Build history of the part. All positions in model axes, mm. A direction names the side the tool comes from. Round coordinates to 2 decimals unless told otherwise and drop trailing zeros. Loops run counter-clockwise (first coordinate to the right, second up) from the corner with the lowest first, then second, coordinate; pieces in that order, holes last. Notation, with made-up numbers: (45.25, 80.25) -> (98.25, 80.25) arc R25 ccw to (98.25, 105.25) -> close; hole circle Ø9 at (68, 74.25). An arc over 180 degrees is marked (long way). Put each result on its own line as item: value. Start each with the question number.
```python
from build123d import *

# Parameters (mm, degrees)
SKETCH1_W           = 25
SKETCH1_H           = 25
BOSS_EXTRUDE1_DEPTH = 15
SKETCH2_R           = 4.3
CUT_EXTRUDE1_DEPTH  = 39.405728739
BOSS_EXTRUDE2_START = 10
SKETCH3_R           = 5.3
SKETCH3_R_2         = 4.3
BOSS_EXTRUDE2_DEPTH = 10
SKETCH4_W           = 15
SKETCH4_H           = 10
CUT_EXTRUDE2_DEPTH  = 28


with BuildPart() as part:
    # Sketch1 → Boss-Extrude1 (new body)
    with BuildSketch(Plane.XY):
        with Locations((12.5, 12.5)):
            Rectangle(SKETCH1_W, SKETCH1_H)
    extrude(amount=BOSS_EXTRUDE1_DEPTH)

    # Sketch2 → Cut-Extrude1 (cut, through all)
    with BuildSketch(Plane.XY.offset(15)):
        with Locations((12.5, 12.5)):
            Circle(SKETCH2_R)
    extrude(amount=-CUT_EXTRUDE1_DEPTH, mode=Mode.SUBTRACT)

    # Sketch3 → Boss-Extrude2 (add)
    with BuildSketch(Plane.XY.offset(15).offset(BOSS_EXTRUDE2_START)):
        with Locations(Location((12.5, 12.5, 0), (0, 0, 180))):
            Circle(SKETCH3_R)
        with Locations((12.5, 12.5)):
            Circle(SKETCH3_R_2, mode=Mode.SUBTRACT)
    extrude(amount=-BOSS_EXTRUDE2_DEPTH)

    # Sketch4 → Cut-Extrude2 (cut)
    with BuildSketch(Plane(origin=(0, 25, 0), x_dir=(1, 0, 0), z_dir=(0, 1, 0))):
        with Locations((12.5, -5)):
            Rectangle(SKETCH4_W, SKETCH4_H)
    extrude(amount=-CUT_EXTRUDE2_DEPTH, mode=Mode.SUBTRACT)


solid = part.part
```
Item 1: Cut at B-B on z = 12.25. Write the cut outline in (x, y), then the cut area to 3 significant figures.
Item 2: Drop flat-ended pins along their axis: pin 1 (2 mm diameter, centred on x = 20.5, y = 14, fed in from -Z); pin 2 (8 mm diameter, centred on x = 3.5, y = 19, fed in from +Z); pin 3 (11 mm diameter, centred on x = 12.5, y = 12.5, fed in from -Z); pin 4 (2 mm diameter, centred on x = 17.5, z = 8.5, fed in from +Y). Give the stop position or say it passes through.
Item 3: Cut at A-A on y = 12.5. Write the cut outline in (x, z).
Item 4: Cut at D-D on z = 7. Write the cut outline in (x, y).
Item 5: Wall check: line 1 (X direction, y = 2.5, z = 8); line 2 (Y direction, x = 12.5, z = 19.75); line 3 (Z direction, x = 22.5, y = 3.25). Give the ranges that are in metal, low to high. Write a range as from..to.
Item 6: Pull direction X, two halves, no side cores. Call faces 4 (the face through (2, 13, 0)), 5 (the face through (25, 12, 7)), 6 (the face through (20, 13, 5)): +X half, -X half, draft (parallel to the pull), parting line (faces both ways), or undercut.
Item 7: Cut at C-C on x = 12.5. Write the cut outline in (y, z).
Item 8: 3-axis set-ups, long thin cutter, end or side, ignore diameter. For faces 1 (the face through (13.649, 17.674, 20.07)), 2 (the face through (5, 13, 5)), 3 (the face through (22, 13, 0)): which of +Z, -Z, +X, -X, +Y, -Y reach the whole face in a straight line?
Ans:
1. outline: (0, 0) -> (25, 0) -> (25, 25) -> (0, 25) -> close; hole circle Ø8.6 at (12.5, 12.5)
1. area: 567 mm2
2. pin 1: stops at z = 0
2. pin 2: stops at z = 15
2. pin 3: stops at z = 10
2. pin 4: passes through
3. outline: (0, 0) -> (5, 0) -> (5, 10) -> (8.2, 10) -> (8.2, 25) -> (7.2, 25) -> (7.2, 15) -> (0, 15) -> close; (16.8, 10) -> (20, 10) -> (20, 0) -> (25, 0) -> (25, 15) -> (17.8, 15) -> (17.8, 25) -> (16.8, 25) -> close
4. outline: (0, 0) -> (5, 0) -> (5, 25) -> (0, 25) -> close; (20, 0) -> (25, 0) -> (25, 25) -> (20, 25) -> close
5. line 1: x = 0..5, 20..25
5. line 2: y = 7.2..8.2, 16.8..17.8
5. line 3: z = 0..15
6. face 4: draft
6. face 5: +X half
6. face 6: undercut
7. outline: (0, 10) -> (8.2, 10) -> (8.2, 25) -> (7.2, 25) -> (7.2, 15) -> (0, 15) -> close; (16.8, 10) -> (25, 10) -> (25, 15) -> (17.8, 15) -> (17.8, 25) -> (16.8, 25) -> close
8. face 1: +Z
8. face 2: -Z, +Y, -Y
8. face 3: -Z, +X, -X, +Y, -Y
